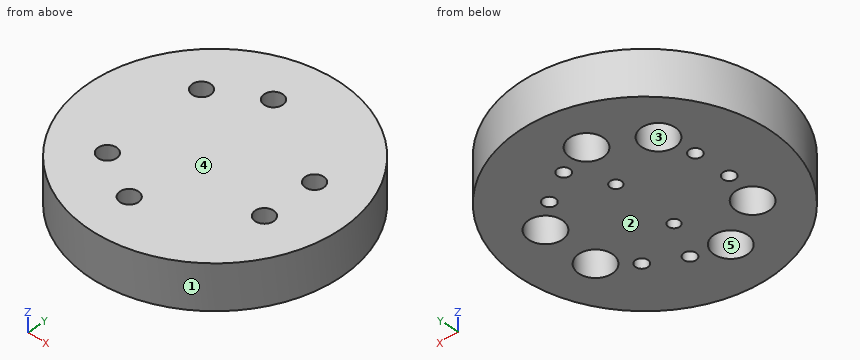
from build123d import *

# Parameters (mm, degrees)
SKETCH_1_R          = 22.5
SKETCH_1_R_2        = 1.65
EXTRUDE_1_DEPTH     = 10
SKETCH_3_R          = 3
CUT_EXTRUDE_1_DEPTH = 7
SKETCH_4_R          = 1.1
CUT_EXTRUDE_2_DEPTH = 8
SKETCH_5_R          = 22.5
SKETCH_5_R_2        = 3
SKETCH_5_R_3        = 1.1
CUT_EXTRUDE_3_DEPTH = 2
SKETCH_6_R          = 1
CUT_EXTRUDE_4_DEPTH = 2


with BuildPart() as part:
    # 스케치1 → 보스-돌출1 (new body)
    with BuildSketch(Plane.XY):
        Circle(SKETCH_1_R)
        with Locations((-2.448439305, 13.885789317)):
            Circle(SKETCH_1_R_2, mode=Mode.SUBTRACT)
        with Locations((-10.801226648, 9.063305297)):
            Circle(SKETCH_1_R_2, mode=Mode.SUBTRACT)
        with Locations((13.249665953, 4.822484021)):
            Circle(SKETCH_1_R_2, mode=Mode.SUBTRACT)
        with Locations((13.249665953, -4.822484021)):
            Circle(SKETCH_1_R_2, mode=Mode.SUBTRACT)
        with Locations((-2.448439305, -13.885789317)):
            Circle(SKETCH_1_R_2, mode=Mode.SUBTRACT)
        with Locations((-10.801226648, -9.063305297)):
            Circle(SKETCH_1_R_2, mode=Mode.SUBTRACT)
    extrude(amount=EXTRUDE_1_DEPTH)

    # 스케치3 → 컷-돌출1 (cut)
    with BuildSketch(Plane(origin=(0, 0, 0), x_dir=(-1, 0, 0), z_dir=(0, 0, -1))):
        with Locations((2.448439305, 13.885789317)):
            Circle(SKETCH_3_R)
        with Locations((10.801226648, 9.063305297)):
            Circle(SKETCH_3_R)
        with Locations((10.801226648, -9.063305297)):
            Circle(SKETCH_3_R)
        with Locations((2.448439305, -13.885789317)):
            Circle(SKETCH_3_R)
        with Locations((-13.249665953, -4.822484021)):
            Circle(SKETCH_3_R)
        with Locations((-13.249665953, 4.822484021)):
            Circle(SKETCH_3_R)
    extrude(amount=-CUT_EXTRUDE_1_DEPTH, mode=Mode.SUBTRACT)

    # 스케치4 → 컷-돌출2 (cut)
    with BuildSketch(Plane(origin=(0, 0, 0), x_dir=(-1, 0, 0), z_dir=(0, 0, -1))):
        with Locations((12.052513913, 3.314650565)):
            Circle(SKETCH_4_R)
        with Locations((12.095108511, -3.155685363)):
            Circle(SKETCH_4_R)
        with Locations((-3.155685363, -12.095108511)):
            Circle(SKETCH_4_R)
        with Locations((-8.780457946, -8.896828551)):
            Circle(SKETCH_4_R)
        with Locations((-8.896828551, 8.780457946)):
            Circle(SKETCH_4_R)
        with Locations((-3.314650565, 12.052513913)):
            Circle(SKETCH_4_R)
    extrude(amount=-CUT_EXTRUDE_2_DEPTH, mode=Mode.SUBTRACT)

    # 스케치5 → 컷-돌출3 (cut)
    with BuildSketch(Plane(origin=(0, 0, 0), x_dir=(-1, 0, 0), z_dir=(0, 0, -1))):
        Circle(SKETCH_5_R)
        with Locations((2.448439305, 13.885789317)):
            Circle(SKETCH_5_R_2, mode=Mode.SUBTRACT)
        with Locations((10.801226648, 9.063305297)):
            Circle(SKETCH_5_R_2, mode=Mode.SUBTRACT)
        with Locations((12.052513913, 3.314650565)):
            Circle(SKETCH_5_R_3, mode=Mode.SUBTRACT)
        with Locations((12.095108511, -3.155685363)):
            Circle(SKETCH_5_R_3, mode=Mode.SUBTRACT)
        with Locations((10.801226648, -9.063305297)):
            Circle(SKETCH_5_R_2, mode=Mode.SUBTRACT)
        with Locations((2.448439305, -13.885789317)):
            Circle(SKETCH_5_R_2, mode=Mode.SUBTRACT)
        with Locations((-3.155685363, -12.095108511)):
            Circle(SKETCH_5_R_3, mode=Mode.SUBTRACT)
        with Locations((-8.780457946, -8.896828551)):
            Circle(SKETCH_5_R_3, mode=Mode.SUBTRACT)
        with Locations((-13.249665953, -4.822484021)):
            Circle(SKETCH_5_R_2, mode=Mode.SUBTRACT)
        with Locations((-13.249665953, 4.822484021)):
            Circle(SKETCH_5_R_2, mode=Mode.SUBTRACT)
        with Locations((-8.896828551, 8.780457946)):
            Circle(SKETCH_5_R_3, mode=Mode.SUBTRACT)
        with Locations((-3.314650565, 12.052513913)):
            Circle(SKETCH_5_R_3, mode=Mode.SUBTRACT)
    extrude(amount=-CUT_EXTRUDE_3_DEPTH, mode=Mode.SUBTRACT)

    # 스케치6 → 컷-돌출4 (cut)
    with BuildSketch(Plane(origin=(0, 0, 2), x_dir=(-1, 0, 0), z_dir=(0, 0, -1))):
        with Locations((0, 5.6)):
            Circle(SKETCH_6_R)
        with Locations((0, -5.6)):
            Circle(SKETCH_6_R)
    extrude(amount=-CUT_EXTRUDE_4_DEPTH, mode=Mode.SUBTRACT)


solid = part.part
Geometry: final body of the model. Coordinates: model frame, mm. Face numbers are marked on the shaded views. A direction names the side the tool comes from. Coordinates: 2 decimals unless noted, no trailing zeros. Write each loop counter-clockwise with the first axis right and the second up, starting at its lowest first coordinate (ties: lowest second). Pieces come first, ordered by that corner, then holes. Notation, with made-up numbers: (-10.75, 24.25) - (37.25, 24.25) arc R22 cw to (37.25, 51.25) - close; hole circle Ø11 at (45.25, 40.25). An arc over 180 degrees is marked (long way). Return JSON: item names as keys, results as strings.
Item 1: Reachability of the marked faces 4 and 5 from +Z, -Z, +X, -X, +Y, -Y: full face, straight path, thin tool, end or side. Return the list, or none.
Completed:
{"face 4": "+Z, +X, -X, +Y, -Y", "face 5": "-Z"}
Item 2: Pull-direction query (Y, two-part tool) for the marked faces 1, 2 and 3; classes: +Y half, -Y half, draft (parallel to the pull), parting line (faces both ways), or undercut.
Completed:
{"face 1": "parting line", "face 2": "draft", "face 3": "undercut"}
Item 3: Section query C-C (z = 5). Count the separate pieces of the cut face and the enclosed holes in it, and give its area (3 significant figures).
Completed:
{"separate pieces": "1", "enclosed holes": "12", "area": "1,400 mm2"}
Item 4: Section query A-A (x = -2.5). Output: boundary loops of the cut face in (y, z).
Completed:
{"outline": "(-22.36, 2) - (-16.89, 2) - (-16.89, 7) - (-15.53, 7) - (-15.53, 10) - (-22.36, 10) - close; (-12.24, 7) - (-10.89, 7) - (-10.89, 2) - (10.89, 2) - (10.89, 7) - (12.24, 7) - (12.24, 10) - (-12.24, 10) - close; (15.53, 7) - (16.89, 7) - (16.89, 2) - (22.36, 2) - (22.36, 10) - (15.53, 10) - close"}
Item 5: Section query B-B (z = 9.25). Output: boundary loops of the cut face in (x, y), and give its area (3 significant figures).
Completed:
{"outline": "circle Ø45 at (0, 0); hole circle Ø3.3 at (-10.8, -9.06); hole circle Ø3.3 at (-10.8, 9.06); hole circle Ø3.3 at (-2.45, -13.89); hole circle Ø3.3 at (-2.45, 13.89); hole circle Ø3.3 at (13.25, -4.82); hole circle Ø3.3 at (13.25, 4.82)", "area": "1,540 mm2"}
Item 6: Section query D-D (y = 18.5). Output: boundary loops of the cut face in (x, z), and give its area (3 significant figures).
Completed:
{"outline": "(-12.81, 2) - (12.81, 2) - (12.81, 10) - (-12.81, 10) - close", "area": "205 mm2"}
Item 7: Pin query (flat end, axial travel): pin 1 Ø3 at (y, z) = (10, 5) entering from +X; pin 2 Ø3 at (y, z) = (13, 4) entering from +X; pin 3 Ø0.7 at (x, y) = (-12.5, 3.5) entering from -Z. Return the tip coordinate at first contact, or that it passes through.
Completed:
{"pin 1": "stops at x = 20.83", "pin 2": "stops at x = 19.34", "pin 3": "stops at z = 8"}
Item 8: Line query: L1, parallel to Y at x = 0, z = 3.2; L2, parallel to X at y = 8, z = 2.75; L3, parallel to X at y = -13, z = 2.5. Output: solid intervals per line, ascending.
Completed:
{"L1": "y = -22.5 to -15.62, -12.15 to -6.6, -4.6 to 4.6, 6.6 to 12.15, 15.62 to 22.5", "L2": "x = -21.03 to -13.61, -8 to 8.12, 9.67 to 21.03", "L3": "x = -18.36 to -5.31, 0.42 to 2.53, 3.78 to 18.36"}
